```python
from build123d import *

# Parameters (mm, degrees)
SCHIZZO1_R                   = 7.5
SCHIZZO1_R_2                 = 2
SCHIZZO1_R_3                 = 8.25
SCHIZZO1_W                   = 3
SCHIZZO1_H                   = 4
ESTRUSIONE_ESTRUSIONE1_DEPTH = 4


with BuildPart() as part:
    # Schizzo1 → Estrusione-Estrusione1 (new body)
    with BuildSketch(Plane.XY):
        Polygon((0, 50), (0, 90), (35, 90), (35, 94), (45, 94), (45, 90), (135, 90), (135, 94), (145, 94), (145, 90), (235, 90), (235, 94), (245, 94), (245, 90), (335, 90), (335, 94), (345, 94), (345, 90), (435, 90), (435, 94), (445, 94), (445, 90), (490, 90), (490, 0), (445, 0), (445, -4), (435, -4), (435, 0), (345, 0), (345, -4), (335, -4), (335, 0), (245, 0), (245, -4), (235, -4), (235, 0), (145, 0), (145, -4), (135, -4), (135, 0), (45, 0), (45, -4), (35, -4), (35, 0), (0, 0), (0, 40), (40, 40), (40, 50), align=None)
        with Locations((457.5, 45)):
            Circle(SCHIZZO1_R, mode=Mode.SUBTRACT)
        with Locations((437.5, 45)):
            Circle(SCHIZZO1_R_2, mode=Mode.SUBTRACT)
        with Locations((467.5, 27.679491924)):
            Circle(SCHIZZO1_R_2, mode=Mode.SUBTRACT)
        with Locations((467.5, 62.320508076)):
            Circle(SCHIZZO1_R_2, mode=Mode.SUBTRACT)
        with Locations((220, 58.25)):
            Circle(SCHIZZO1_R_3, mode=Mode.SUBTRACT)
        with Locations((220, 31.75)):
            Circle(SCHIZZO1_R_3, mode=Mode.SUBTRACT)
        Polygon((50, 77.928932188), (50, 12.071067812), (82.928932188, 45), align=None, mode=Mode.SUBTRACT)
        Polygon((130, 77.928932188), (130, 12.071067812), (97.071067812, 45), align=None, mode=Mode.SUBTRACT)
        Polygon((57.071067812, 85), (90, 52.071067812), (122.928932188, 85), align=None, mode=Mode.SUBTRACT)
        Polygon((123.1448388, 4.784093388), (57.077189669, 5.006121857), (90, 37.928932188), align=None, mode=Mode.SUBTRACT)
        Polygon((150, 77.928932188), (150, 12.071067812), (182.928932188, 45), align=None, mode=Mode.SUBTRACT)
        Polygon((157.071067812, 85), (190, 52.071067812), (222.928932188, 85), align=None, mode=Mode.SUBTRACT)
        Polygon((223.1448388, 4.784093388), (157.077189669, 5.006121857), (190, 37.928932188), align=None, mode=Mode.SUBTRACT)
        Polygon((250, 77.928932188), (250, 12.071067812), (282.928932188, 45), align=None, mode=Mode.SUBTRACT)
        Polygon((330, 77.928932188), (330, 12.071067812), (297.071067812, 45), align=None, mode=Mode.SUBTRACT)
        Polygon((257.071067812, 85), (290, 52.071067812), (322.928932188, 85), align=None, mode=Mode.SUBTRACT)
        Polygon((323.1448388, 4.784093388), (257.077189669, 5.006121857), (290, 37.928932188), align=None, mode=Mode.SUBTRACT)
        Polygon((350, 77.928932188), (350, 12.071067812), (382.928932188, 45), align=None, mode=Mode.SUBTRACT)
        Polygon((430, 77.928932188), (430, 12.071067812), (397.071067812, 45), align=None, mode=Mode.SUBTRACT)
        Polygon((357.071067812, 85), (390, 52.071067812), (422.928932188, 85), align=None, mode=Mode.SUBTRACT)
        Polygon((423.1448388, 4.784093388), (357.077189669, 5.006121857), (390, 37.928932188), align=None, mode=Mode.SUBTRACT)
        with Locations((24.5, 67)):
            Rectangle(SCHIZZO1_W, SCHIZZO1_H, mode=Mode.SUBTRACT)
        Polygon((206.75, 54.678932188), (197.071067812, 45), (206.75, 35.321067812), align=None, mode=Mode.SUBTRACT)
    extrude(amount=ESTRUSIONE_ESTRUSIONE1_DEPTH)


solid = part.part
```
Read the model definition and answer for the solid it produces. Units are mm, in the model's axes. A direction names the side the tool comes from. Round coordinates to 2 decimals unless told otherwise and drop trailing zeros. Write each loop counter-clockwise with the first axis right and the second up, starting at its lowest first coordinate (ties: lowest second). Pieces come first, ordered by that corner, then holes. Notation, with made-up numbers: (63, 2) -> (94, 2) arc R21 cw to (94, 38) -> close; hole circle Ø2 at (70, 58.25). An arc over 180 degrees is marked (long way). Answer in a Markdown table with one row per item. Add a question column.
1) Given P1, Ø1.2, axis at x = 463, z = 2.5, coming from the +Y side, flat-ended and moving along its own axis, determine where the tip first touches the part or whether it passes through.
2) Find section C-C, the plane z = 0.8. State how many separate pieces and enclosed holes the cut face has, and give its area (3 significant figures).
3) Which of the six approach directions +Z, -Z, +X, -X, +Y, -Y give full straight-line access (tool end or side, diameter ignored) to faces 1 (the face through (248, 46, 4)), 2 (the face through (173.305, 68.766, 1.972))?
4) Find section B-B, the plane x = 406. Determine the outline of the cut face in (y, z), and give its area (3 significant figures).
5) Consider line 1 (Y direction, x = 213, z = 3.1); line 2 (Y direction, x = 406, z = 3.3); line 3 (X direction, y = 81, z = 3.3). Determine where each line is inside the solid, lowest interval first.
6) Find section A-A, the plane x = 457.5. Determine the outline of the cut face in (y, z).
7) Find section D-D, the plane x = 308. Determine the outline of the cut face in (y, z), and give its area (3 significant figures).
8) Determine the mould class of faces 3 (the face through (201.84, 40.23, 1.97)), 4 (the face through (248, 46, 0)) for opening direction Y: pulls with the +Y half, pulls with the -Y half, needs draft (parallel to the pull), parting line crosses it, or undercut.
Findings below:
| question | item | result |
|---|---|---|
| 1 | P1 | y = 90 |
| 2 | separate pieces | 1 |
| 2 | enclosed holes | 23 |
| 2 | area | 27,100 mm² |
| 3 | face 1 | +Z, +X, -X, +Y, -Y |
| 3 | face 2 | +Z, -Z |
| 4 | outline | (0, 0) -> (4.84, 0) -> (4.84, 4) -> (0, 4) -> close; (21.93, 0) -> (36.07, 0) -> (36.07, 4) -> (21.93, 4) -> close; (53.93, 0) -> (68.07, 0) -> (68.07, 4) -> (53.93, 4) -> close; (85, 0) -> (90, 0) -> (90, 4) -> (85, 4) -> close |
| 4 | area | 153 mm² |
| 5 | line 1 | 0 to 4.82, 14.93 to 27.38, 36.12 to 53.88, 62.62 to 75.07, 85 to 90 |
| 5 | line 2 | 0 to 4.84, 21.93 to 36.07, 53.93 to 68.07, 85 to 90 |
| 5 | line 3 | 0 to 61.07, 118.93 to 161.07, 218.93 to 261.07, 318.93 to 361.07, 418.93 to 490 |
| 6 | outline | (0, 0) -> (37.5, 0) -> (37.5, 4) -> (0, 4) -> close; (52.5, 0) -> (90, 0) -> (90, 4) -> (52.5, 4) -> close |
| 7 | outline | (0, 0) -> (4.83, 0) -> (4.83, 4) -> (0, 4) -> close; (19.93, 0) -> (34.07, 0) -> (34.07, 4) -> (19.93, 4) -> close; (55.93, 0) -> (70.07, 0) -> (70.07, 4) -> (55.93, 4) -> close; (85, 0) -> (90, 0) -> (90, 4) -> (85, 4) -> close |
| 7 | area | 152 mm² |
| 8 | face 3 | undercut |
| 8 | face 4 | needs draft |
